Build history of the part. All positions in model axes, mm. Face numbers are marked on the shaded views. A direction names the side the tool comes from. Give positions to 0.01 mm unless a question says otherwise; leave off trailing zeros. Order: outer loops, then holes, each group sorted by start corner. A loop starts at its lowest first (then second) coordinate and runs counter-clockwise, first axis right, second up. Notation, with made-up numbers: (11.25, 86.5) -> (50.25, 86.5) arc R13 ccw to (50.25, 98.5) -> close; hole circle Ø9 at (56.5, 62). An arc over 180 degrees is marked (long way). Use a Markdown table: item, result. Add a question column.
Autodesk Inventor part; units mm, degrees
ref_plane "YZ Plane" through (0, 0, 0) normal (1, 0, 0) x (0, 1, 0)
ref_plane "XZ Plane" through (0, 0, 0) normal (0, 1, 0) x (-1, 0, 0)
ref_plane "XY Plane" through (0, 0, 0) normal (0, 0, 1) x (1, 0, 0)
sketch "Skizze1" plane through (0, 0, 0) normal (0, 0, 1) x (1, 0, 0)
  line L0 (0, -14.25) -> (0, 14.25) construction
  arc A0 (-5.5, -14.25) -> (5.5, -14.25) centre (0, -14.25) ccw
  arc A1 (5.5, 14.25) -> (-5.5, 14.25) centre (0, 14.25) ccw
  line L1 (0, 28.35) -> (0, -28.35) construction
  line L2 (-16.45, 0) -> (16.45, 0) construction
  circle A2 centre (0, 14.25) radius 1.5
  circle A3 centre (0, -14.25) radius 1.5
  circle A4 centre (0, 14.25) radius 6 construction
  circle A5 centre (0, -14.25) radius 6 construction
  line L3 (0, 20.25) -> (0, -20.25) construction
  circle A6 centre (0, 14.25) radius 3
  circle A7 centre (0, -14.25) radius 3
  circle A8 centre (0, 0) radius 9.75
  line L4 (-5.5, 14.25) -> (-5.5, 10.3833)
  line L5 (-5.5, -10.3833) -> (-5.5, -14.25)
  line L6 (5.5, -14.25) -> (5.5, -10.3833)
  line L7 (5.5, 10.3833) -> (5.5, 14.25)
  arc A9 (5.5, -10.3833) -> (5.5, 10.3833) centre (0, 0) ccw
  arc A10 (-5.5, 10.3833) -> (-5.5, -10.3833) centre (0, 0) ccw
  circle A11 centre (0, 0) radius 6.35 construction
  circle A12 centre (-4.4901, 4.4901) radius 1.5
  circle A13 centre (-4.4901, -4.4901) radius 1.5
  circle A14 centre (4.4901, -4.4901) radius 1.5
  circle A15 centre (4.4901, 4.4901) radius 1.5
  line L8 (-4.4901, 4.4901) -> (0, 0) construction
  dimension "d4" = 12
  dimension "d31" = 12.7
  dimension "d1" = 3
  dimension "d2" = 4
  dimension "d5" = 40.5
  dimension "d19" = 1.5
  dimension "d26" = 19.5
  dimension "d28" = 2
  dimension "d32" = 3
  dimension "d35" = 360
  dimension "d37" = 45
extrude "Extrusion1" add sketch "Skizze1" against normal blind 7 contours L5 A10 L4 A1 L7 A9 L6 A0 | A6 | A7
chamfer "Fase2" distance 2 distance2 7 6 edges at (5.5, -12.3166, 0) (0, -19.75, 0) (-5.5, -12.3166, 0) (0, 19.75, 0) (5.5, 12.3166, 0) (-5.5, 12.3166, 0) measured on face at (4.1094, 12.7287, 0)
extrude "Extrusion4" add sketch "Skizze1" against normal blind 0.5 from surface at -7 contours A6 | A7
extrude "Extrusion6" add sketch "Skizze1" along normal blind 2 from surface at -7 contours A8
properties part number "HarmonicDrive-WaveGenerator-Bottom"
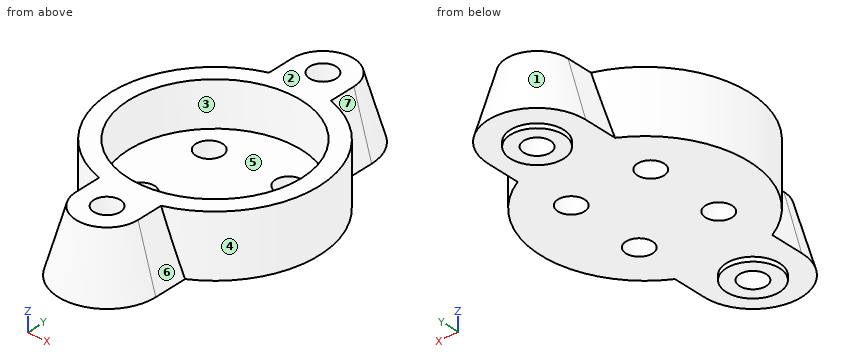
(1) Mould opens along Y. For the marked faces 1, 2 and 3 say: released by +Y, released by -Y, zero draft, split by the parting line, or undercut.
(2) Band-saw the part on B-B on y = 0. Give the cut face in (x, z), plus the area to 3 significant figures.
(3) Pin check, flat tips, straight feed: pin 1 Ø4 at (x, y) = (-3, -11.5) entering from -Z; pin 2 Ø12 at (x, y) = (-2.5, 1.5) entering from -Z; pin 3 Ø2.5 at (x, y) = (0, -14.25) entering from -Z; pin 4 Ø1 at (x, z) = (9, -2.5) entering from +Y. Stop position of each tip, or through.
(4) Band-saw the part on C-C on z = -2.25. Give the cut face in (x, y).
(5) Wall check: probe 1 along Y at (x, z) = (1, -0.75); probe 2 along X at (y, z) = (3.5, -6); probe 3 along Y at (x, z) = (3.25, -3.5). Give the ranges that are in metal, low to high.
(6) Tool access for the marked faces 4, 5, 6 and 7: list every direction of +Z, -Z, +X, -X, +Y, -Y with a clear straight run to the whole face (end or side of a thin tool).
(7) Band-saw the part on A-A on x = 0. State how many separate pieces and enclosed holes the cut face has, plus the area to 3 significant figures.
(8) Band-saw the part on D-D on y = 4. Give the cut face in (x, z).
Response:
| question | item | result |
|---|---|---|
| 1 | face 1 | released by +Y |
| 1 | face 2 | zero draft |
| 1 | face 3 | undercut |
| 2 | outline | (-11.75, -7) -> (11.75, -7) -> (11.75, 0) -> (9.75, 0) -> (9.75, -5) -> (-9.75, -5) -> (-9.75, 0) -> (-11.75, 0) -> close |
| 2 | area | 67.0 mm² |
| 3 | pin 1 | stops at z = -7.5 |
| 3 | pin 2 | stops at z = -7 |
| 3 | pin 3 | passes through |
| 3 | pin 4 | stops at y = 8.11 |
| 4 | outline | (-4.14, -14.25) arc R4.14 ccw to (4.14, -14.25) -> (4.14, -11) arc R11.75 ccw to (4.14, 11) -> (4.14, 14.25) arc R4.14 ccw to (-4.14, 14.25) -> (-4.14, 11) arc R11.75 ccw to (-4.14, -11) -> close; hole circle Ø19.5 at (0, 0); hole circle Ø3 at (0, -14.25); hole circle Ø3 at (0, 14.25) |
| 5 | probe 1 | y = -17.83 to -15.37, -13.13 to -9.7, 9.7 to 13.13, 15.37 to 17.83 |
| 5 | probe 2 | x = -11.22 to -5.62, -3.36 to 3.36, 5.62 to 11.22 |
| 5 | probe 3 | y = -17.36 to -9.19, 9.19 to 17.36 |
| 6 | face 4 | +Z, +X |
| 6 | face 5 | +Z |
| 6 | face 6 | +Z, +X, -Y |
| 6 | face 7 | +Z, +X, +Y |
| 7 | separate pieces | 3 |
| 7 | enclosed holes | 0 |
| 7 | area | 126 mm² |
| 8 | outline | (-11.05, -7) -> (-5.91, -7) -> (-5.91, -5) -> (-8.89, -5) -> (-8.89, 0) -> (-11.05, 0) -> close; (-3.07, -7) -> (3.07, -7) -> (3.07, -5) -> (-3.07, -5) -> close; (5.91, -7) -> (11.05, -7) -> (11.05, 0) -> (8.89, 0) -> (8.89, -5) -> (5.91, -5) -> close |
